For this review, take the finished solid that the model builds, in its own axes (mm). Round coordinates to 2 decimals unless told otherwise and drop trailing zeros. Order: outer loops, then holes, each group sorted by start corner. A loop starts at its lowest first (then second) coordinate and runs counter-clockwise, first axis right, second up. Notation, with made-up numbers: M -32.5,-27.75 L 7.5,-27.75 A21 cw 7.5,-17.75 Z; hole C -39.5,-12 d5. An arc over 180 degrees is marked long. Use a Markdown table: item, result.
Autodesk Inventor part; units mm, degrees
ref_plane "YZ Plane" through (0, 0, 0) normal (1, 0, 0) x (0, 1, 0)
ref_plane "XZ Plane" through (0, 0, 0) normal (0, 1, 0) x (-1, 0, 0)
ref_plane "XY Plane" through (0, 0, 0) normal (0, 0, 1) x (1, 0, 0)
sketch "스케치1" plane through (0, 0, 0) normal (0, 0, 1) x (1, 0, 0)
  line L0 (0, 0) -> (-36, 0)
  line L1 (0, 0) -> (36, 0) construction
  line L2 (-36, 0) -> (-36, 6)
  line L3 (-36, 0) -> (-36, -6)
  line L4 (-36, 0) -> (-30, 0) construction
  line L5 (0, 0) -> (36, 0)
  line L6 (0, 0) -> (36, 0) construction
  line L7 (36, 0) -> (36, 6)
  line L8 (36, 0) -> (36, -6)
  line L9 (36, 0) -> (42, 0) construction
  line L10 (-36, -6) -> (36, -6)
  line L11 (-36, 6) -> (36, 6)
  circle A0 centre (-30, 0) radius 4.025
  circle A1 centre (30, 0) radius 4.025
  dimension "d0" = 36
  dimension "d1" = 180
  dimension "d2" = 6
  dimension "d3" = 90
  dimension "d4" = 6
  dimension "d5" = 90
  dimension "d6" = 0
  dimension "d7" = 36
  dimension "d8" = 6
  dimension "d9" = 6
  dimension "d10" = 90
  dimension "d11" = 8.05
  dimension "d12" = 8.05
  dimension "d13" = 6
  dimension "d14" = 6
  dimension "d15" = 30
  dimension "d16" = 30
extrude "돌출1" add sketch "스케치1" along normal blind 4 contours L5 A1 L8 L10 L3 L0 A0 | L0 A0 L2 L11 L7 L5 A1
fillet "모깎기1" radius 6 2 edges at (36, -6, 2) (36, 6, 2)
fillet "모깎기2" radius 6 2 edges at (-36, -6, 2) (-36, 6, 2)
sketch "스케치4" plane through (0, 0, 0) normal (0, 0, -1) x (-1, 0, 0)
  circle A0 centre (30, 0) radius 4.025
  circle A1 centre (30, 0) radius 4.8
  point P0 (0, 0)
  dimension "d27" = 9.6
sketch "스케치5" plane through (0, 0, 0) normal (0, 0, -1) x (-1, 0, 0)
  circle A0 centre (30, 0) radius 4.8
  arc A1 (30, -6) -> (30, 6) centre (30, 0) ccw
  line L0 (30, 6) -> (-30, 6)
  arc A2 (-30, 6) -> (-30, -6) centre (-30, 0) ccw
  line L1 (-30, -6) -> (30, -6)
  circle A3 centre (-30, 0) radius 4.035
  circle A4 centre (-30, 0) radius 4.8
  point P0 (0, 0)
properties part number "Link" material "알루미늄 6061"
Q1. Add section B-B (y = -1.25). Write out the cut boundary in (x, z).
Determined:
| item | result |
|---|---|
| outline | M -35.87,0 L -33.83,0 L -33.83,4 L -35.87,4 Z; M -26.17,0 L 26.17,0 L 26.17,4 L -26.17,4 Z; M 33.83,0 L 35.87,0 L 35.87,4 L 33.83,4 Z |
Q2. Draft analysis for pull direction Y (two halves, no side actions). For faces 1 (the cylindrical face through (-34.02, -0.18, 1.97)), 2 (the flat face through (0, -6, 2)), 3 (the flat face through (-1, 0, 4)), state which applies: pulls with the +Y half, pulls with the -Y half, needs draft (parallel to the pull), parting line crosses it, or undercut.
Determined:
| item | result |
|---|---|
| face 1 | undercut |
| face 2 | pulls with the -Y half |
| face 3 | needs draft |
Q3. Add section A-A (z = 3.2). Give the number of separate pieces and of enclosed holes in the cut face, then the cut area to 3 significant figures.
Determined:
| item | result |
|---|---|
| separate pieces | 1 |
| enclosed holes | 2 |
| area | 731 mm^2 |
Q4. Wall thickness on line 1 along X through (y, z) = (0, 1.1) (3 decimals); line 2 along Y through (x, z) = (-30, 2.1) (3 decimals); line 3 along X through (y, z) = (-1.5, 3.55): over which ranges is each line inside the solid? List them lowest first. Write a range as [from, to].
Determined:
| item | result |
|---|---|
| line 1 | x = [-36, -34.025], [-25.975, 25.975], [34.025, 36] |
| line 2 | y = [-6, -4.025], [4.025, 6] |
| line 3 | x = [-35.81, -33.74], [-26.26, 26.26], [33.74, 35.81] |
Q5. Clearance check with a flat-ended pin moving along its axis: pin 1 (1 mm diameter, centred on y = -3, z = 3, fed in from -X). State where the tip first meets the part, or that it passes through.
Determined:
| item | result |
|---|---|
| pin 1 | stops at x = -35.45 |
